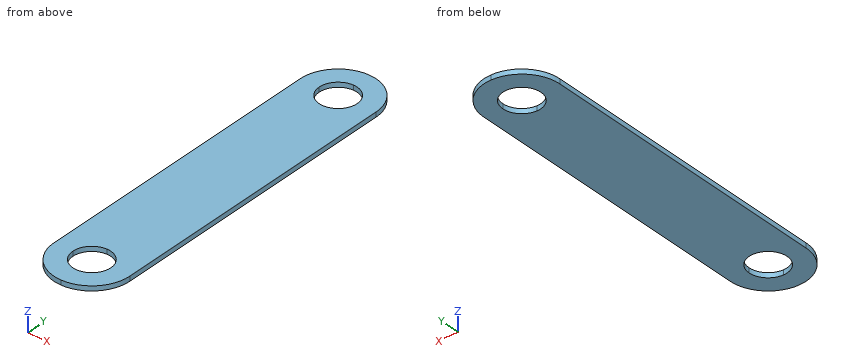
from build123d import *

# Parameters (mm, degrees)
F1_DEPTH = 1.5875


with BuildPart() as f1:
    # F0 (on Top) → F1 (new body)
    with BuildSketch(Plane.XY):
        with BuildLine():
            ThreePointArc((0, 57.15), (4.490128, 55.290128), (6.35, 50.8))
            Line((6.35, 50.8), (12.7, 50.8))
            ThreePointArc((12.7, 50.8), (8.980256, 59.780256), (0, 63.5))
            Line((0, 63.5), (0, 57.15))
        make_face()
        with BuildLine():
            Line((12.7, 50.8), (6.35, 50.8))
            ThreePointArc((6.35, 50.8), (4.490128, 46.309872), (0, 44.45))
            Line((0, 44.45), (0, -44.45))
            ThreePointArc((0, -44.45), (4.490128, -46.309872), (6.35, -50.8))
            Line((6.35, -50.8), (12.7, -50.8))
            Line((12.7, -50.8), (12.7, 50.8))
        make_face()
        with BuildLine():
            ThreePointArc((-6.35, 50.8), (-4.490128, 55.290128), (0, 57.15))
            Line((0, 57.15), (0, 63.5))
            ThreePointArc((0, 63.5), (-8.980256, 59.780256), (-12.7, 50.8))
            Line((-12.7, 50.8), (-6.35, 50.8))
        make_face()
        with BuildLine():
            Line((0, -44.45), (0, 44.45))
            ThreePointArc((0, 44.45), (-4.490128, 46.309872), (-6.35, 50.8))
            Line((-6.35, 50.8), (-12.7, 50.8))
            Line((-12.7, 50.8), (-12.7, -50.8))
            Line((-12.7, -50.8), (-6.35, -50.8))
            ThreePointArc((-6.35, -50.8), (-4.490128, -46.309872), (0, -44.45))
        make_face()
        with BuildLine():
            ThreePointArc((0, -63.5), (8.980256, -59.780256), (12.7, -50.8))
            Line((12.7, -50.8), (6.35, -50.8))
            ThreePointArc((6.35, -50.8), (4.490128, -55.290128), (0, -57.15))
            Line((0, -57.15), (0, -63.5))
        make_face()
        with BuildLine():
            ThreePointArc((-12.7, -50.8), (-8.980256, -59.780256), (0, -63.5))
            Line((0, -63.5), (0, -57.15))
            ThreePointArc((0, -57.15), (-4.490128, -55.290128), (-6.35, -50.8))
            Line((-6.35, -50.8), (-12.7, -50.8))
        make_face()
    extrude(amount=F1_DEPTH)


solid = f1.part
The listing builds one solid part. Answer for the finished solid, in the listing's coordinates (mm). Coordinates: 2 decimals unless noted, no trailing zeros. Write each loop counter-clockwise with the first axis right and the second up, starting at its lowest first coordinate (ties: lowest second). Pieces come first, ordered by that corner, then holes. Notation, with made-up numbers: (-24, 73.25) - (24, 73.25) arc R35 cw to (24, 106.25) - close; hole circle Ø4 at (59.25, 64). An arc over 180 degrees is marked (long way). Answer as CSV lines item,"result".
1. Find section A-A (y = -48). Give the vertices of the cut face in (x, z).
Computed values:
outline,"(-12.7, 0) - (-5.7, 0) - (-5.7, 1.59) - (-12.7, 1.59) - close; (5.7, 0) - (12.7, 0) - (12.7, 1.59) - (5.7, 1.59) - close"
2. Find section C-C (z = 1.2). Give the vertices of the cut face in (x, y).
Computed values:
outline,"(-12.7, -50.8) arc R12.7 ccw to (12.7, -50.8) - (12.7, 50.8) arc R12.7 ccw to (-12.7, 50.8) - close; hole circle Ø12.7 at (0, -50.8); hole circle Ø12.7 at (0, 50.8)"
3. Find section D-D (y = 45.5). Give the vertices of the cut face in (x, z).
Computed values:
outline,"(-12.7, 0) - (-3.5, 0) - (-3.5, 1.59) - (-12.7, 1.59) - close; (3.5, 0) - (12.7, 0) - (12.7, 1.59) - (3.5, 1.59) - close"
4. Straight lines are drawn through the part: line 1 (Y direction, x = 5.75, z = 0.75); line 2 (Y direction, x = -5.5, z = 0.8); line 3 (X direction, y = -55, z = 1.1). For each, find the intervals that lie inside material, in ascending order. Write a range as [from, to].
Computed values:
line 1,"y = [-62.12, -53.49], [-48.11, 48.11], [53.49, 62.12]"
line 2,"y = [-62.25, -53.97], [-47.63, 47.63], [53.97, 62.25]"
line 3,"x = [-11.99, -4.76], [4.76, 11.99]"
5. Find section B-B (x = 2). Give the vertices of the cut face in (y, z).
Computed values:
outline,"(-63.34, 0) - (-56.83, 0) - (-56.83, 1.59) - (-63.34, 1.59) - close; (-44.77, 0) - (44.77, 0) - (44.77, 1.59) - (-44.77, 1.59) - close; (56.83, 0) - (63.34, 0) - (63.34, 1.59) - (56.83, 1.59) - close"
